Check sheet for the modelled part. Datum: model origin and axes. Units: mm. A direction names the side the tool comes from. Coordinates: 2 decimals unless noted, no trailing zeros. Loops run counter-clockwise (first coordinate to the right, second up) from the corner with the lowest first, then second, coordinate; pieces in that order, holes last. Notation, with made-up numbers: (-28.75, -34) - (18.25, -34) arc R17 cw to (18.25, -18) - close; hole circle Ø4 at (38.5, -32). An arc over 180 degrees is marked (long way). Write each question's results on one line, items separated by ' | '. Start each with the question number.
1. Gauge pin test, flat end, axial feed: P1, Ø1, axis at y = -1, z = 11.5, coming from the -X side. Record the tip position at first contact, or that the pin passes through.
2. Cross-section at C-C (y = -0.5). Record the cut outline in (x, z).
3. Cross-section at D-D (z = 9.25). Give the number of separate pieces and of enclosed holes in the cut face, and give its area (3 significant figures).
4. Thickness scan on line 1 (Y direction, x = -0.5, z = 5); line 2 (X direction, y = 0.5, z = 14); line 3 (Z direction, x = 17.5, y = 1). Record the ranges inside material, lowest first. Write a range as [from, to].
5. Cross-section at B-B (z = 13.5). Record the cut outline in (x, y), and give its area (3 significant figures).
6. Tool access check on faces 4 (the face through (0.567, 1.525, 15.715)), 5 (the face through (10.214, -3, 8)), 6 (the face through (0.861, -7.076, 0.285)). Record the directions out of +Z, -Z, +X, -X, +Y, -Y that give a thin tool (end or side, any length) a straight path to the whole face; none if there is none.
7. Draft check along Y on faces 1 (the face through (-2, -6.775, 7)), 2 (the face through (16, -3, 0)), 3 (the face through (13.882, 0.676, 6.204)). Enter one of: released by +Y, released by -Y, zero draft, split by the parting line, or undercut.
8. Cross-section at A-A (x = 9). Record the cut outline in (y, z).
```python
from build123d import *

# Parameters (mm, degrees)
F0_W     = 36
F0_H     = 14
F1_DEPTH = 16
F2_W     = 20
F2_H     = 8
F2_W_2   = 30.9440002977
F3_DEPTH = 29.3
F4_R     = 4.875
F5_DEPTH = 11
F5_TAPER = 3
F6_R     = 4.875
F7_DEPTH = 11
F7_TAPER = 3
F8_R     = 1
F4_R_2   = 2.25
F9_DEPTH = 16


with BuildPart() as f1:
    # F0 (on Top) → F1 (new body)
    with BuildSketch(Plane.XY):
        with Locations((8.2136405466, -2.7754378021)):
            Rectangle(F0_W, F0_H)
    extrude(amount=F1_DEPTH)

    # F2 (on face) → F3 (cut, symmetric)
    with BuildSketch(Plane.XY.offset(16)):
        with Locations((0.2136405466, -2.7754378021)):
            Rectangle(F2_W, F2_H)
        with Locations((-25.2583596023, -2.7754378021)):
            Rectangle(F2_W_2, F2_H)
    extrude(amount=F3_DEPTH, both=True, mode=Mode.SUBTRACT)

    # F4 (on face) → F5 (cut)
    with BuildSketch(Plane(origin=(0, 4.2245621979, 0), x_dir=(-1, 0, 0), z_dir=(0, 1, 0))):
        with Locations((-18.2136405466, 8)):
            Circle(F4_R)
    extrude(amount=-F5_DEPTH, taper=F5_TAPER, mode=Mode.SUBTRACT)

    # F6 (on face) → F7 (cut)
    with BuildSketch(Plane.XZ.offset(9.7754378021)):
        with Locations((18.2136405466, 8)):
            Circle(F6_R)
    extrude(amount=-F7_DEPTH, taper=F7_TAPER, mode=Mode.SUBTRACT)

    # F8
    f8_edges = [f1.edges().sort_by_distance(p)[0] for p in [
        (26.213641, -9.775438, 8),
        (26.213641, 4.224562, 8),
        (26.213641, -2.775438, 0),
        (26.213641, -2.775438, 16),
        (8.213641, -9.775438, 16),
        (-9.786359, -8.275438, 16),
        (0.213641, -6.775438, 16),
        (10.213641, -2.775438, 16),
        (0.213641, 1.224562, 16),
        (-9.786359, 2.724562, 16),
        (8.213641, 4.224562, 16),
        (8.213641, -9.775438, 0),
        (-9.786359, -8.275438, 0),
        (0.213641, -6.775438, 0),
        (10.213641, -2.775438, 0),
        (0.213641, 1.224562, 0),
        (-9.786359, 2.724562, 0),
        (8.213641, 4.224562, 0),
        (-9.786359, 4.224562, 8),
        (-9.786359, -9.775438, 8),
    ]]
    fillet(f8_edges, radius=F8_R)

    # F4 (on face) → F9 (cut, symmetric)
    with BuildSketch(Plane(origin=(0, 4.2245621979, 0), x_dir=(-1, 0, 0), z_dir=(0, 1, 0))):
        with Locations((-0.2136405466, 8)):
            Circle(F4_R_2)
    extrude(amount=F9_DEPTH, both=True, mode=Mode.SUBTRACT)


solid = f1.part
```
Established:
1) P1: x = 10.21
2) outline: (10.21, 1) arc R1 ccw to (11.21, 0) - (25.21, 0) arc R1 ccw to (26.21, 1) - (26.21, 15) arc R1 ccw to (25.21, 16) - (11.21, 16) arc R1 ccw to (10.21, 15) - close; hole circle Ø9.25 at (18.21, 8)
3) separate pieces: 4 | enclosed holes: 0 | area: 194 mm^2
4) line 1: [-9.78, -6.78], [1.22, 4.22] | line 2: [10.21, 26.21] | line 3: [0, 3.35], [12.65, 16]
5) outline: (-9.79, -8.78) arc R1 ccw to (-8.79, -9.78) - (25.21, -9.78) arc R1 ccw to (26.21, -8.78) - (26.21, 3.22) arc R1 ccw to (25.21, 4.22) - (-8.79, 4.22) arc R1 ccw to (-9.79, 3.22) - (-9.79, 1.22) - (10.21, 1.22) - (10.21, -6.78) - (-9.79, -6.78) - close | area: 343 mm^2
6) face 4: +Z, -X | face 5: +Z, -Z, -X | face 6: -Z, -X
7) face 1: undercut | face 2: zero draft | face 3: released by +Y
8) outline: (-9.78, 1) arc R1 ccw to (-8.78, 0) - (-7.78, 0) arc R1 ccw to (-6.78, 1) - (-6.78, 15) arc R1 ccw to (-7.78, 16) - (-8.78, 16) arc R1 ccw to (-9.78, 15) - close; (1.22, 1) arc R1 ccw to (2.22, 0) - (3.22, 0) arc R1 ccw to (4.22, 1) - (4.22, 15) arc R1 ccw to (3.22, 16) - (2.22, 16) arc R1 ccw to (1.22, 15) - close
